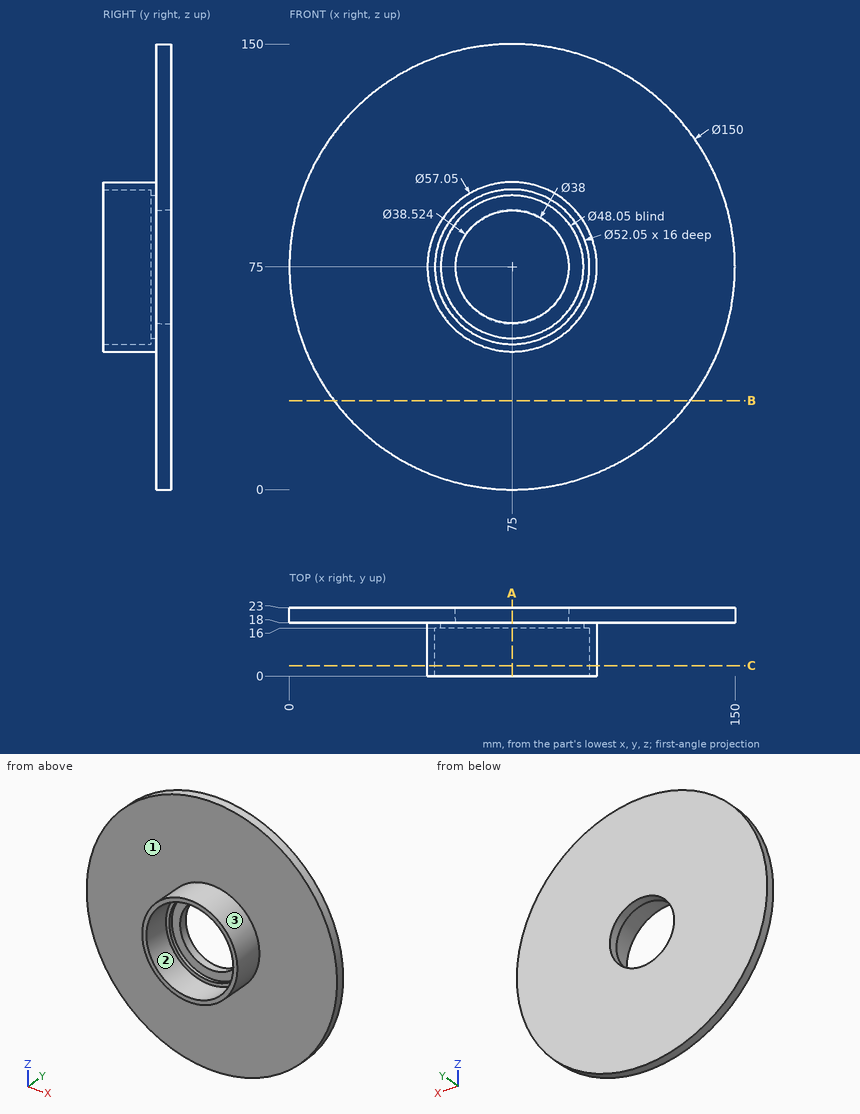
Check sheet for the drawn part. Datum: minimum x, y, z corner. Units: mm. Round coordinates to 2 decimals unless told otherwise and drop trailing zeros. Loops run counter-clockwise (first coordinate to the right, second up) from the corner with the lowest first, then second, coordinate; pieces in that order, holes last. Notation, with made-up numbers: (-15.75, 13.5) - (35.25, 13.5) arc R16 ccw to (35.25, 36.5) - close; hole circle Ø3 at (27, 22.25). An arc over 180 degrees is marked (long way). Write item = value, one per line. Start each with the question number.
1. Section check B-B on z = 30. Enter the section's corners in (x, y).
2. Mould release check, pull along X, two halves, no side actions. Record for the marked faces 1, 2 and 3: released by +X, released by -X, zero draft, split by the parting line, or undercut.
3. Section check C-C on y = 3.5. Enter the section's corners in (x, z) (3 decimals).
4. Thickness scan on line 1 (Z direction, x = 75, y = 7) (3 decimals); line 2 (Z direction, x = 75, y = 16.95) (3 decimals); line 3 (Y direction, x = 35.5, z = 13). Record the ranges inside material, lowest first.
5. Section check A-A on x = 75. Enter the section's corners in (y, z) (3 decimals), then the cut area to 3 significant figures.
6. Depth check by flat-ended pin: pin 1 (2 mm diameter, centred on x = 81, z = 36.5, fed in from -Y); pin 2 (5 mm diameter, centred on x = 77.5, y = 8.5, fed in from +Z) (3 decimals); pin 3 (4 mm diameter, centred on y = 18.5, z = 19, fed in from +X). Enter the tip coordinate at first touch or a pass-through.
Working result:
q1.outline = (15, 18) - (135, 18) - (135, 23) - (15, 23) - close
q2.face_1 = zero draft
q2.face_2 = undercut
q2.face_3 = split by the parting line
q3.outline = circle Ø57.05 at (75, 75); hole circle Ø52.05 at (75, 75)
q4.line_1 = 46.475 to 48.975, 101.025 to 103.525
q4.line_2 = 46.475 to 50.975, 99.025 to 103.525
q4.line_3 = 18 to 23
q5.outline = (0, 46.475) - (18, 46.475) - (18, 0) - (23, 0) - (23, 55.738) - (18, 56) - (18, 50.975) - (16, 50.975) - (16, 48.975) - (0, 48.975) - close; (0, 101.025) - (16, 101.025) - (16, 99.025) - (18, 99.025) - (18, 94) - (23, 94.262) - (23, 150) - (18, 150) - (18, 103.525) - (0, 103.525) - close
q5.area = 657 mm^2
q6.pin_1 = 18
q6.pin_2 = 103.525
q6.pin_3 = 127.05
